Read the model definition and answer for the solid it produces. Units are mm, in the model's axes. Face numbers are marked on the shaded views. Coordinates: 2 decimals unless noted, no trailing zeros. Order: outer loops, then holes, each group sorted by start corner. A loop starts at its lowest first (then second) coordinate and runs counter-clockwise, first axis right, second up. Notation, with made-up numbers: (7.25, 48.5) -> (49.25, 48.5) arc R35 ccw to (49.25, 80.5) -> close; hole circle Ø6 at (8, 1.5). An arc over 180 degrees is marked (long way). Return JSON: item names as keys, results as strings. Group by question number.
```python
from build123d import *

# Parameters (mm, degrees)
SKETCH2_W           = 184
SKETCH2_H           = 135
BOSS_EXTRUDE1_DEPTH = 2
SKETCH3_W           = 184
SKETCH3_H           = 135
SKETCH3_W_2         = 160
SKETCH3_H_2         = 125
BOSS_EXTRUDE2_DEPTH = 1
BOSS_EXTRUDE3_DEPTH = 2
CUT_EXTRUDE1_REACH  = 170.88
SKETCH5_R           = 2.25


with BuildPart() as part:
    # Sketch2 → Boss-Extrude1 (new body)
    with BuildSketch(Plane(origin=(0, 0, 0), x_dir=(1, 0, 0), z_dir=(0, 1, 0))):
        with Locations((62.722752399, 0)):
            Rectangle(SKETCH2_W, SKETCH2_H)
        with BuildLine():
            Line((4.722752399, 55.5), (119.722752399, 55.5))
            ThreePointArc((119.722752399, 55.5), (126.79382021, 52.571067812), (129.722752399, 45.5))
            Line((129.722752399, 45.5), (129.722752399, -45.5))
            ThreePointArc((129.722752399, -45.5), (126.79382021, -52.571067812), (119.722752399, -55.5))
            Line((119.722752399, -55.5), (4.722752399, -55.5))
            ThreePointArc((4.722752399, -55.5), (-2.348315413, -52.571067812), (-5.277247601, -45.5))
            Line((-5.277247601, -45.5), (-5.277247601, 45.5))
            ThreePointArc((-5.277247601, 45.5), (-2.348315413, 52.571067812), (4.722752399, 55.5))
        make_face(mode=Mode.SUBTRACT)
    extrude(amount=BOSS_EXTRUDE1_DEPTH)

    # Sketch3 → Boss-Extrude2 (add)
    with BuildSketch(Plane(origin=(0, 2, 0), x_dir=(1, 0, 0), z_dir=(0, 1, 0))):
        with Locations((62.722752399, 0)):
            Rectangle(SKETCH3_W, SKETCH3_H)
        with Locations((62.722752399, 0)):
            Rectangle(SKETCH3_W_2, SKETCH3_H_2, mode=Mode.SUBTRACT)
    extrude(amount=BOSS_EXTRUDE2_DEPTH)

    # Sketch4 → Boss-Extrude3 (add)
    with BuildSketch(Plane(origin=(0, 3, 0), x_dir=(1, 0, 0), z_dir=(0, 1, 0))):
        Polygon((154.722752399, 67.5), (-29.277247601, 67.5), (-29.277247601, 66.5), (153.722752399, 66.5), (153.722752399, -66.5), (-29.277247601, -66.5), (-29.277247601, -67.5), (154.722752399, -67.5), align=None)
    extrude(amount=BOSS_EXTRUDE3_DEPTH)

    # Sketch5 → Cut-Extrude1 (cut, up to next)
    with BuildSketch(Plane.XZ, mode=Mode.PRIVATE) as cut_extrude1_sk1:
        with Locations(Location((-23.277247601, 60.5, 0), (0, 0, 270))):
            Circle(SKETCH5_R)
    cut_extrude1_tool1 = extrude(cut_extrude1_sk1.sketch, amount=-CUT_EXTRUDE1_REACH, mode=Mode.PRIVATE) & part.part
    # Sketch5 → Cut-Extrude1 (cut, up to next)
    with BuildSketch(Plane.XZ, mode=Mode.PRIVATE) as cut_extrude1_sk2:
        with Locations(Location((-23.277247601, -60.5, 0), (0, 0, 270))):
            Circle(SKETCH5_R)
    cut_extrude1_tool2 = extrude(cut_extrude1_sk2.sketch, amount=-CUT_EXTRUDE1_REACH, mode=Mode.PRIVATE) & part.part
    # Sketch5 → Cut-Extrude1 (cut, up to next)
    with BuildSketch(Plane.XZ, mode=Mode.PRIVATE) as cut_extrude1_sk3:
        with Locations(Location((147.722752399, -60.5, 0), (0, 0, 270))):
            Circle(SKETCH5_R)
    cut_extrude1_tool3 = extrude(cut_extrude1_sk3.sketch, amount=-CUT_EXTRUDE1_REACH, mode=Mode.PRIVATE) & part.part
    # Sketch5 → Cut-Extrude1 (cut, up to next)
    with BuildSketch(Plane.XZ, mode=Mode.PRIVATE) as cut_extrude1_sk4:
        with Locations(Location((147.722752399, 60.5, 0), (0, 0, 270))):
            Circle(SKETCH5_R)
    cut_extrude1_tool4 = extrude(cut_extrude1_sk4.sketch, amount=-CUT_EXTRUDE1_REACH, mode=Mode.PRIVATE) & part.part
    add(cut_extrude1_tool1.solids().sort_by_distance((-23.277248, 0, 60.5))[0], mode=Mode.SUBTRACT)
    add(cut_extrude1_tool2.solids().sort_by_distance((-23.277248, 0, -60.5))[0], mode=Mode.SUBTRACT)
    add(cut_extrude1_tool3.solids().sort_by_distance((147.722752, 0, -60.5))[0], mode=Mode.SUBTRACT)
    add(cut_extrude1_tool4.solids().sort_by_distance((147.722752, 0, 60.5))[0], mode=Mode.SUBTRACT)


solid = part.part
```
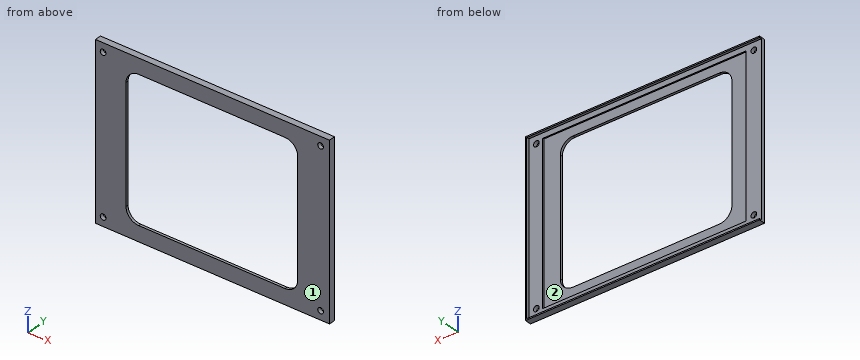
1. Find section A-A on x = 76. Determine the outline of the cut face in (y, z).
2. For a pull along X with two mould halves and no side action, classify the marked faces 1 and 2 as released by +X, released by -X, zero draft, split by the parting line, or undercut.
3. Find section C-C on z = -21.5. Determine the outline of the cut face in (x, y).
4. Find section B-B on z = -60.5. Determine the outline of the cut face in (x, y), and give its area (3 significant figures).
5. Straight lines are drawn through the part: L1, parallel to X at y = 2.15, z = 60.5; L2, parallel to X at y = 0.7, z = -60.5; L3, parallel to Z at x = 99, y = 1.8. For each, find the intervals that lie inside material, in ascending order.
6. Find section D-D on x = 134. Determine the outline of the cut face in (y, z), and give its area (3 significant figures).
7. Given pin 1 (0.6 mm diameter, centred on y = 3.5, z = -17.5, fed in from -X); pin 2 (6 mm diameter, centred on x = -23.28, z = -60.5, fed in from +Y), each flat-ended and moving along its own axis, determine where each tip first touches the part or whether it passes through.
Result:
{
 "1": {"outline": "(0, -67.5) -> (5, -67.5) -> (5, -66.5) -> (3, -66.5) -> (3, -62.5) -> (2, -62.5) -> (2, -55.5) -> (0, -55.5) -> close; (0, 55.5) -> (2, 55.5) -> (2, 62.5) -> (3, 62.5) -> (3, 66.5) -> (5, 66.5) -> (5, 67.5) -> (0, 67.5) -> close"},
 "2": {"face 1": "zero draft", "face 2": "undercut"},
 "3": {"outline": "(-29.28, 0) -> (-5.28, 0) -> (-5.28, 2) -> (-17.28, 2) -> (-17.28, 3) -> (-29.28, 3) -> close; (129.72, 0) -> (154.72, 0) -> (154.72, 5) -> (153.72, 5) -> (153.72, 3) -> (142.72, 3) -> (142.72, 2) -> (129.72, 2) -> close"},
 "4": {"outline": "(-29.28, 0) -> (-25.53, 0) -> (-25.53, 3) -> (-29.28, 3) -> close; (-21.03, 0) -> (145.47, 0) -> (145.47, 3) -> (142.72, 3) -> (142.72, 2) -> (-17.28, 2) -> (-17.28, 3) -> (-21.03, 3) -> close; (149.97, 0) -> (154.72, 0) -> (154.72, 5) -> (153.72, 5) -> (153.72, 3) -> (149.97, 3) -> close", "area": "367 mm^2"},
 "5": {"L1": "-29.28 to -25.53, -21.03 to -17.28, 142.72 to 145.47, 149.97 to 154.72", "L2": "-29.28 to -25.53, -21.03 to 145.47, 149.97 to 154.72", "L3": "-67.5 to -55.5, 55.5 to 67.5"},
 "6": {"outline": "(0, -67.5) -> (5, -67.5) -> (5, -66.5) -> (3, -66.5) -> (3, -62.5) -> (2, -62.5) -> (2, 62.5) -> (3, 62.5) -> (3, 66.5) -> (5, 66.5) -> (5, 67.5) -> (0, 67.5) -> close", "area": "284 mm^2"},
 "7": {"pin 1": "x = 153.72", "pin 2": "y = 3"}
}
